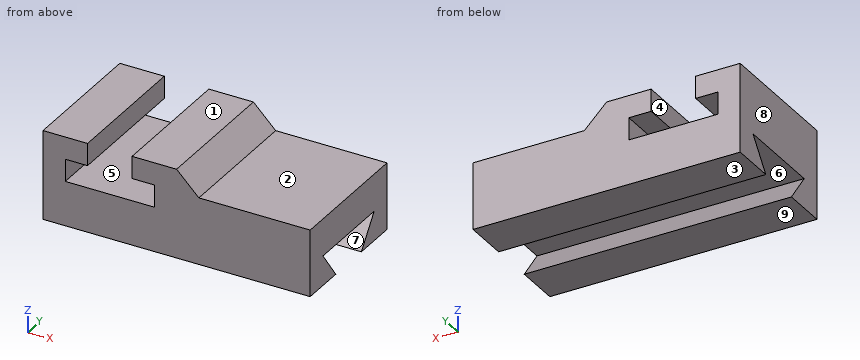
from build123d import *

# Parameters (mm, degrees)
F1_DEPTH = 76.2
F3_DEPTH = 152.4
F5_DEPTH = 152.4
F7_DEPTH = 152.4


with BuildPart() as f1:
    # F0 (on Front) → F1 (new body)
    with BuildSketch(Plane.XZ):
        Polygon((152.4, 38.1), (88.9, 38.1), (76.2, 50.8), (50.8, 50.8), (50.8, 38.1), (63.5, 38.1), (63.5, 25.4), (12.7, 25.4), (12.7, 38.1), (25.4, 38.1), (25.4, 50.8), (0, 50.8), (0, 0), (152.4, 0), align=None)
    extrude(amount=-F1_DEPTH)

    # F2 (on Right) → F3 (join)
    with BuildSketch(Plane.YZ):
        Polygon((12.7, 12.7), (25.4, 0), (50.8, 0), (63.5, 12.7), align=None)
    extrude(amount=F3_DEPTH)

    # F4 (on face) → F5 (join)
    with BuildSketch(Plane.YZ.offset(152.4)):
        Polygon((12.7, 11.3952), (25.4, 0), (50.8, 0), (63.5, 11.3952), align=None)
    extrude(amount=-F5_DEPTH)

    # F6 (on face) → F7 (cut)
    with BuildSketch(Plane.YZ.offset(152.4)):
        Polygon((12.7, 16.891001), (25.4, 0), (50.8, 0), (63.5, 16.891001), align=None)
    extrude(amount=-F7_DEPTH, mode=Mode.SUBTRACT)


solid = f1.part
The listing builds one solid part. Answer for the finished solid, in the listing's coordinates (mm). Face numbers are marked on the shaded views. A direction names the side the tool comes from. Give positions to 0.01 mm unless a question says otherwise; leave off trailing zeros. Write each loop counter-clockwise with the first axis right and the second up, starting at its lowest first coordinate (ties: lowest second). Pieces come first, ordered by that corner, then holes. Notation, with made-up numbers: (63.5, 62.5) - (120.5, 62.5) arc R14 cw to (120.5, 81.5) - close; hole circle Ø7 at (-2.5, 13.25). An arc over 180 degrees is marked (long way). Use a Markdown table: item, result.
1. Section A-A on z = 42.5 is taken. Write down the section's boundary in (x, y), plus the area to 3 significant figures.
Values follow:
| item | result |
|---|---|
| outline | (0, 0) - (25.4, 0) - (25.4, 76.2) - (0, 76.2) - close; (50.8, 0) - (84.5, 0) - (84.5, 76.2) - (50.8, 76.2) - close |
| area | 4,500 mm² |
2. A tool of negligible diameter and unlimited length cuts with its end or side. For the marked faces 1, 2, 3, 4 and 5, from which of +Z, -Z, +X, -X, +Y, -Y can it reach the whole face along a straight path? Write none if from no direction.
Values follow:
| item | result |
|---|---|
| face 1 | +Z, +X, -X, +Y, -Y |
| face 2 | +Z, +X, +Y, -Y |
| face 3 | -Z, +X, -X, +Y, -Y |
| face 4 | +Z, +Y, -Y |
| face 5 | +Y, -Y |
3. Section B-B on x = 72 is taken. Write down the section's boundary in (y, z).
Values follow:
| item | result |
|---|---|
| outline | (0, 0) - (25.4, 0) - (12.7, 16.89) - (63.5, 16.89) - (50.8, 0) - (76.2, 0) - (76.2, 50.8) - (0, 50.8) - close |
4. Each of these flat-tipped pins is pushed along its axis until it touches: P1, Ø2, axis at x = 111.5, z = 22.5, coming from the -Y side; P2, Ø4, axis at x = 67.5, y = 36, coming from the -Z side; P3, Ø4, axis at y = 38.5, z = 47.5, coming from the +X side; P4, Ø12, axis at x = 98.5, y = 30, coming from the +Z side. Where does it stop, or does it pass through?
Values follow:
| item | result |
|---|---|
| P1 | stops at y = 0 |
| P2 | stops at z = 16.89 |
| P3 | stops at x = 81.5 |
| P4 | stops at z = 38.1 |
5. Section D-D on y = 22 is taken. Write down the section's boundary in (x, z).
Values follow:
| item | result |
|---|---|
| outline | (0, 0) - (152.4, 0) - (152.4, 4.52) - (0, 4.52) - close; (0, 16.89) - (152.4, 16.89) - (152.4, 38.1) - (88.9, 38.1) - (76.2, 50.8) - (50.8, 50.8) - (50.8, 38.1) - (63.5, 38.1) - (63.5, 25.4) - (12.7, 25.4) - (12.7, 38.1) - (25.4, 38.1) - (25.4, 50.8) - (0, 50.8) - close |
6. Section C-C on y = 66.5 is taken. Write down the section's boundary in (x, z), plus the area to 3 significant figures.
Values follow:
| item | result |
|---|---|
| outline | (0, 0) - (152.4, 0) - (152.4, 38.1) - (88.9, 38.1) - (76.2, 50.8) - (50.8, 50.8) - (50.8, 38.1) - (63.5, 38.1) - (63.5, 25.4) - (12.7, 25.4) - (12.7, 38.1) - (25.4, 38.1) - (25.4, 50.8) - (0, 50.8) - close |
| area | 5,890 mm² |
7. Find the intervals of material crossed by probe 1 along X at (y, z) = (72, 31); probe 2 along Z at (x, y) = (52.5, 27); probe 3 along Z at (x, y) = (100.5, 69), in increasing order. Write a range as from..to.
Values follow:
| item | result |
|---|---|
| probe 1 | x = 0..12.7, 63.5..152.4 |
| probe 2 | z = 16.89..25.4, 38.1..50.8 |
| probe 3 | z = 0..38.1 |
8. For a pull along Z with two mould halves and no side action, classify the marked faces 6, 7, 8 and 9 as released by +Z, released by -Z, zero draft, split by the parting line, or undercut.
Values follow:
| item | result |
|---|---|
| face 6 | undercut |
| face 7 | undercut |
| face 8 | zero draft |
| face 9 | released by -Z |
